from build123d import *

# Parameters (mm, degrees)
F1_DEPTH = 25
F2_DEPTH = 12


# Not quite as in the source:
# - a feature names something its author has since deleted; it is built from what else it names


with BuildPart() as f1:
    # F0 (on Front) → F1 (new body)
    with BuildSketch(Plane.XZ):
        with BuildLine():
            Line((-44.8163774249, 23.8675290289), (-41.9426736004, 23.8675290289))
            ThreePointArc((-41.9426736004, 23.8675290289), (-45.7285804931, 26.6455290289), (-49.5144873857, 23.8675290289))
            Line((-49.5144873857, 23.8675290289), (-46.6407835612, 23.8675290289))
            ThreePointArc((-46.6407835612, 23.8675290289), (-45.7285804931, 24.1767790289), (-44.8163774249, 23.8675290289))
        make_face()
        with BuildLine():
            Line((-46.6407835612, 23.8675290289), (-44.8163774249, 23.8675290289))
            ThreePointArc((-44.8163774249, 23.8675290289), (-45.7285804931, 24.1767790289), (-46.6407835612, 23.8675290289))
        make_face()
    extrude(amount=F1_DEPTH)



with BuildPart() as f1b:
    # F0 (on Front) → F1, piece 2 (new body)
    with BuildSketch(Plane.XZ):
        with BuildLine():
            ThreePointArc((-49.5144873857, 21.4860290289), (-45.7285804931, 18.7080290289), (-41.9426736004, 21.4860290289))
            Line((-41.9426736004, 21.4860290289), (-44.8163774249, 21.4860290289))
            ThreePointArc((-44.8163774249, 21.4860290289), (-45.7285804931, 21.1767790289), (-46.6407835612, 21.4860290289))
            Line((-46.6407835612, 21.4860290289), (-49.5144873857, 21.4860290289))
        make_face()
        with BuildLine():
            ThreePointArc((-46.6407835612, 21.4860290289), (-45.7285804931, 21.1767790289), (-44.8163774249, 21.4860290289))
            Line((-44.8163774249, 21.4860290289), (-46.6407835612, 21.4860290289))
        make_face()
    extrude(amount=F1_DEPTH)


with BuildPart() as f1_1:
    add(f1.part)

    add(f1b.part)  # F2 merges F1b
    # F0 (on Front) → F2 (join)
    with BuildSketch(Plane.XZ):
        with BuildLine():
            Line((-46.6407835612, 23.8675290289), (-49.5144873857, 23.8675290289))
            ThreePointArc((-49.5144873857, 23.8675290289), (-49.6973304931, 22.6767790289), (-49.5144873857, 21.4860290289))
            Line((-49.5144873857, 21.4860290289), (-46.6407835612, 21.4860290289))
            ThreePointArc((-46.6407835612, 21.4860290289), (-47.2285804931, 22.6767790289), (-46.6407835612, 23.8675290289))
        make_face()
        with BuildLine():
            ThreePointArc((-41.9426736004, 21.4860290289), (-41.8058075872, 22.0744259007), (-41.7598304931, 22.6767790289))
            ThreePointArc((-41.7598304931, 22.6767790289), (-41.8058075872, 23.2791321571), (-41.9426736004, 23.8675290289))
            Line((-41.9426736004, 23.8675290289), (-44.8163774249, 23.8675290289))
            ThreePointArc((-44.8163774249, 23.8675290289), (-44.3835331701, 23.3407426566), (-44.2285804931, 22.6767790289))
            ThreePointArc((-44.2285804931, 22.6767790289), (-44.3835331701, 22.0128154012), (-44.8163774249, 21.4860290289))
            Line((-44.8163774249, 21.4860290289), (-41.9426736004, 21.4860290289))
        make_face()
    extrude(amount=F2_DEPTH)


solid = f1_1.part
Check sheet for the modelled part. Datum: model origin and axes. Units: mm. A direction names the side the tool comes from. Round coordinates to 2 decimals unless told otherwise and drop trailing zeros. Order: outer loops, then holes, each group sorted by start corner. A loop starts at its lowest first (then second) coordinate and runs counter-clockwise, first axis right, second up.
(1) Go/stop test with a flat-tipped pin: P1, Ø1.2, axis at x = -43, z = 22.5, coming from the -Y side. Record where the tip stops, or that it passes through.
(2) Access from +Z, -Z, +X, -X, +Y, -Y to the whole of each face (thin tool, end or side, straight path). Record for faces 3 (the flat face through (-46, -15, 21.486)), 4 (the flat face through (-46, -25, 25)), 5 (the cylindrical face through (-47.23, -5.92, 22.66)), 6 (the flat face through (-49, -12, 23)).
(3) Cross-section at A-A, the plane y = -6. Enter the section's corners in (x, z).
(4) Scan lines: probe 1 along X at (y, z) = (-1.5, 22.5); probe 2 along Z at (x, y) = (-44.5, -12.25); probe 3 along Y at (x, z) = (-48.25, 23.5). Record each from-to range of solid material in increasing order.
(5) Cross-section at D-D, the plane y = -16.5. Enter the section's corners in (x, z), and give its area (3 significant figures).
(6) Draft check along X on faces 1 (the flat face through (-43, -12, 23)), 2 (the flat face through (-46, -15, 23.868)). Enter one of: pulls with the +X half, pulls with the -X half, needs draft (parallel to the pull), parting line crosses it, or undercut.
(7) Cross-section at B-B, the plane z = 23. Enter the section's corners in (x, y), and give its area (3 significant figures).
(8) Cross-section at C-C, the plane x = -48. Enter the section's corners in (y, z).
Check sheet entries:
1. P1: stops at y = -12
2. face 3: -Y
2. face 4: +Z, -Z, +X, -X, -Y
2. face 5: +Y, -Y
2. face 6: +X, -X, -Y
3. outline: circle Ø7.94 at (-45.73, 22.68); hole (-46.64, 21.49) - (-44.82, 21.49) arc R1.5 ccw to (-44.82, 23.87) - (-46.64, 23.87) arc R1.5 ccw to start
4. probe 1: x = -49.69 to -47.22, -44.24 to -41.76
4. probe 2: z = 18.9 to 21.49, 23.87 to 26.45
4. probe 3: y = -12 to 0
5. outline: (-49.51, 21.49) arc R3.97 ccw to (-41.94, 21.49) - close; (-49.51, 23.87) - (-41.94, 23.87) arc R3.97 ccw to start
5. area: 30.9 mm2
6. face 1: needs draft
6. face 2: undercut
7. outline: (-49.68, -12) - (-47.19, -12) - (-47.19, 0) - (-49.68, 0) - close; (-44.26, -12) - (-41.77, -12) - (-41.77, 0) - (-44.26, 0) - close
7. area: 59.8 mm2
8. outline: (-25, 19.42) - (0, 19.42) - (0, 25.93) - (-25, 25.93) - (-25, 23.87) - (-12, 23.87) - (-12, 21.49) - (-25, 21.49) - close
